Can you work these out from the model? Positions are in its coordinate system, mm. Face numbers are marked on the shaded views. Coordinates: 2 decimals unless noted, no trailing zeros. Loops run counter-clockwise (first coordinate to the right, second up) from the corner with the lowest first, then second, coordinate; pieces in that order, holes last.
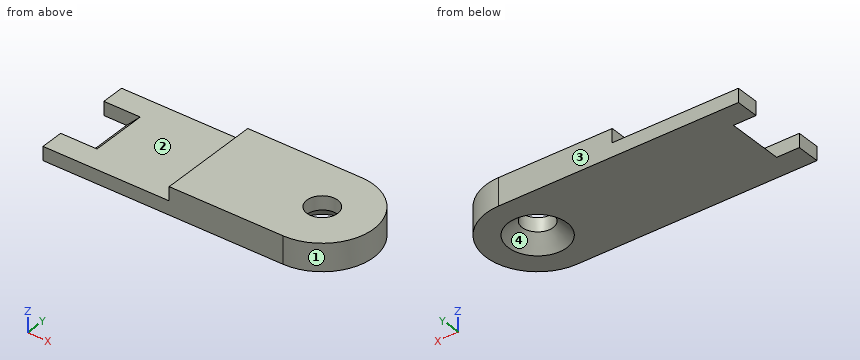
```python
from build123d import *

# Parameters (mm, degrees)
F0_R     = 2.25
F1_DEPTH = 4
F2_DEPTH = 2
F3_SIZE  = 1.99999


# Not quite as in the source:
# - a fillet or chamfer is up to 0.001 mm smaller than in the source, because OpenCascade refuses the exact size


with BuildPart() as f1:
    # F0 (on Top) → F1 (new body)
    with BuildSketch(Plane.XY):
        with BuildLine():
            Line((14, 7.5), (-2.6, 7.5))
            Line((-2.6, 7.5), (-2.6, -7.5))
            Line((-2.6, -7.5), (14, -7.5))
            ThreePointArc((14, -7.5), (21.5, 0), (14, 7.5))
        make_face()
        with Locations((14, 0)):
            Circle(F0_R, mode=Mode.SUBTRACT)
    extrude(amount=F1_DEPTH)

    # F0 (on Top) → F2 (join)
    with BuildSketch(Plane.XY):
        Polygon((-2.6, 7.5), (-21, 7.5), (-21, 4.125), (-17.7, 4.125), (-17.7, -4.125), (-21, -4.125), (-21, -7.5), (-2.6, -7.5), align=None)
    extrude(amount=F2_DEPTH)

    # F3 (size 2 in the source; OpenCascade refuses exactly that, so slightly less here)
    f3_edges = [f1.edges().sort_by_distance(p)[0] for p in [
        (11.75, 0, 0),
        (-17.7, 0, 2),
    ]]
    chamfer(f3_edges, length=F3_SIZE)


solid = f1.part
```
Item 1: Suppose I cut it at B-B, the plane z = 1.5. Please give me the cut outline in (x, y) (3 decimals).
Results are:
outline: (-21, -7.5) - (14, -7.5) arc R7.5 ccw to (14, 7.5) - (-21, 7.5) - (-21, 4.125) - (-16.2, 4.125) - (-16.2, -4.125) - (-21, -4.125) - close; hole circle Ø5.5 at (14, 0)
Item 2: Suppose I cut it at C-C, the plane x = -12. Please give me the cut outline in (y, z), plus the area to 3 significant figures.
Results are:
outline: (-7.5, 0) - (7.5, 0) - (7.5, 2) - (-7.5, 2) - close
area: 30.0 mm2
Item 3: I'm going to push flat-ended pins straight in: P1, Ø0.6, axis at y = -3.5, z = 3.5, coming from the -X side; P2, Ø6, axis at x = 14, y = 0, coming from the -Z side; P3, Ø1.5, axis at y = 2, z = 2, coming from the +X side. Where does each tip first touch, or does it pass through?
Results are:
P1: stops at x = -2.6
P2: stops at z = 1.25
P3: stops at x = 21.4
Item 4: Suppose I cut it at D-D, the plane y = 6.5. Please give me the cut outline in (x, z), plus the area to 3 significant figures.
Results are:
outline: (-21, 0) - (17.74, 0) - (17.74, 4) - (-2.6, 4) - (-2.6, 2) - (-21, 2) - close
area: 118 mm2
Item 5: I need wall thicknesses on line 1 along Y through (x, z) = (14, 2.85); line 2 along Z through (x, y) = (-9, -4.75); line 3 along X through (y, z) = (-0.75, 1.9). Which ranges of each line are inside material? Lowest first, please.
Results are:
line 1: y = -7.5 to -2.25, 2.25 to 7.5
line 2: z = 0 to 2
line 3: x = -15.8 to 11.77, 16.23 to 21.46
Item 6: We'd pull the mould along Y, two halves only. Please class the marked faces 1, 2, 3 and 4: +Y half, -Y half, draft (parallel to the pull), parting line (faces both ways), or undercut.
Results are:
face 1: parting line
face 2: draft
face 3: +Y half
face 4: undercut
